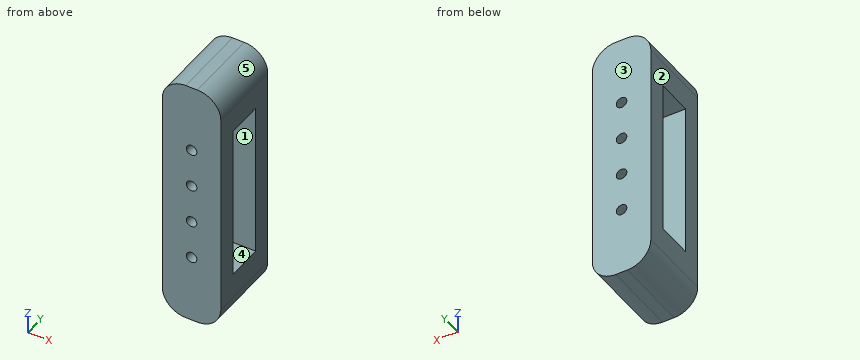
```python
from build123d import *

# Parameters (mm, degrees)
SKETCH1_W           = 15
SKETCH1_H           = 65
SKETCH1_R           = 1.35
BOSS_EXTRUDE1_DEPTH = 19.5
FILLET1_R           = 6
SKETCH2_W           = 40
SKETCH2_H           = 9.5
CUT_EXTRUDE1_DEPTH  = 20


with BuildPart() as part:
    # Sketch1 → Boss-Extrude1 (new body)
    with BuildSketch(Plane(origin=(0, 0, 0), x_dir=(1, 0, 0), z_dir=(0, 1, 0))):
        with Locations((0, -32.5)):
            Rectangle(SKETCH1_W, SKETCH1_H)
        with Locations((0, -17.5)):
            Circle(SKETCH1_R, mode=Mode.SUBTRACT)
        with Locations((0, -27.5)):
            Circle(SKETCH1_R, mode=Mode.SUBTRACT)
        with Locations((0, -37.5)):
            Circle(SKETCH1_R, mode=Mode.SUBTRACT)
        with Locations((0, -47.5)):
            Circle(SKETCH1_R, mode=Mode.SUBTRACT)
    extrude(amount=BOSS_EXTRUDE1_DEPTH)

    # Fillet1
    fillet1_edges = [part.edges().sort_by_distance(p)[0] for p in [
        (-7.5, 9.75, 0),
        (7.5, 9.75, 0),
        (7.5, 9.75, 65),
        (-7.5, 9.75, 65),
    ]]
    fillet(fillet1_edges, radius=FILLET1_R)

    # Sketch2 → Cut-Extrude1 (cut)
    with BuildSketch(Plane.ZY.offset(7.5)):
        with Locations((32.5, 9.75)):
            Rectangle(SKETCH2_W, SKETCH2_H)
    extrude(amount=-CUT_EXTRUDE1_DEPTH, mode=Mode.SUBTRACT)


solid = part.part
```
Source: CAD feature listing. Evaluate the final solid. Frame: model axes, mm. Face numbers are marked on the shaded views. A direction names the side the tool comes from. Give positions to 0.01 mm unless a question says otherwise; leave off trailing zeros. Order: outer loops, then holes, each group sorted by start corner. A loop starts at its lowest first (then second) coordinate and runs counter-clockwise, first axis right, second up. Notation, with made-up numbers: (89, 32.5) -> (116, 32.5) arc R15 cw to (116, 41.5) -> close; hole circle Ø2 at (17.5, -11.75). An arc over 180 degrees is marked (long way). Use a Markdown table: item, result.
Q1. Section D-D (z = 27.5). Return the cut outline in (x, y), and give its area (3 significant figures).
A:
| item | result |
|---|---|
| outline | (-7.5, 0) -> (-1.35, 0) -> (-1.35, 5) -> (-7.5, 5) -> close; (-7.5, 14.5) -> (-1.35, 14.5) -> (-1.35, 19.5) -> (-7.5, 19.5) -> close; (1.35, 0) -> (7.5, 0) -> (7.5, 5) -> (1.35, 5) -> close; (1.35, 14.5) -> (7.5, 14.5) -> (7.5, 19.5) -> (1.35, 19.5) -> close |
| area | 123 mm^2 |
Q2. Section B-B (y = 13.5). Return the cut outline in (x, z).
A:
| item | result |
|---|---|
| outline | (-7.5, 6) arc R6 ccw to (-1.5, 0) -> (1.5, 0) arc R6 ccw to (7.5, 6) -> (7.5, 12.5) -> (-7.5, 12.5) -> close; (-7.5, 52.5) -> (7.5, 52.5) -> (7.5, 59) arc R6 ccw to (1.5, 65) -> (-1.5, 65) arc R6 ccw to (-7.5, 59) -> close |
Q3. Section A-A (z = 20). Return the cut outline in (x, y), and give its area (3 significant figures).
A:
| item | result |
|---|---|
| outline | (-7.5, 0) -> (7.5, 0) -> (7.5, 5) -> (-7.5, 5) -> close; (-7.5, 14.5) -> (7.5, 14.5) -> (7.5, 19.5) -> (-7.5, 19.5) -> close |
| area | 150 mm^2 |
Q4. Access query for the marked faces 1 and 2. Directions: +Z, -Z, +X, -X, +Y, -Y. A direction counts if a zero-diameter tool reaches every point of the face in a straight line with its end or side. Return the directions, or none.
A:
| item | result |
|---|---|
| face 1 | +X, -X |
| face 2 | +Z, -Z, -X, +Y, -Y |
Q5. First-contact query: P1, Ø2, axis at x = 4, y = 10, coming from the -Z side; P2, Ø1.5, axis at x = 2.5, y = 16, coming from the -Z side; P3, Ø1.5, axis at x = 4, y = 14.5, coming from the +Z side. Flat tips, straight axial feed; report the tip coordinate or a pass-through.
A:
| item | result |
|---|---|
| P1 | z = 0.19 |
| P2 | z = 0.01 |
| P3 | z = 64.74 |
Q6. Section C-C (y = 1.75). Return the cut outline in (x, z).
A:
| item | result |
|---|---|
| outline | (-7.5, 6) arc R6 ccw to (-1.5, 0) -> (1.5, 0) arc R6 ccw to (7.5, 6) -> (7.5, 59) arc R6 ccw to (1.5, 65) -> (-1.5, 65) arc R6 ccw to (-7.5, 59) -> close; hole circle Ø2.7 at (0, 17.5); hole circle Ø2.7 at (0, 27.5); hole circle Ø2.7 at (0, 37.5); hole circle Ø2.7 at (0, 47.5) |
Q7. Pull-direction query (Z, two-part tool) for the marked faces 3, 4 and 5; classes: +Z half, -Z half, draft (parallel to the pull), parting line (faces both ways), or undercut.
A:
| item | result |
|---|---|
| face 3 | draft |
| face 4 | undercut |
| face 5 | +Z half |
Q8. Material intervals for line 1 (Z direction, x = 0, y = 2.8); line 2 (X direction, y = 2.8, z = 47.5); line 3 (Y direction, x = -3.75, z = 34.5), sorted ascending. Write a range as [from, to].
A:
| item | result |
|---|---|
| line 1 | [0, 16.15], [18.85, 26.15], [28.85, 36.15], [38.85, 46.15], [48.85, 65] |
| line 2 | [-7.5, -1.35], [1.35, 7.5] |
| line 3 | [0, 5], [14.5, 19.5] |
